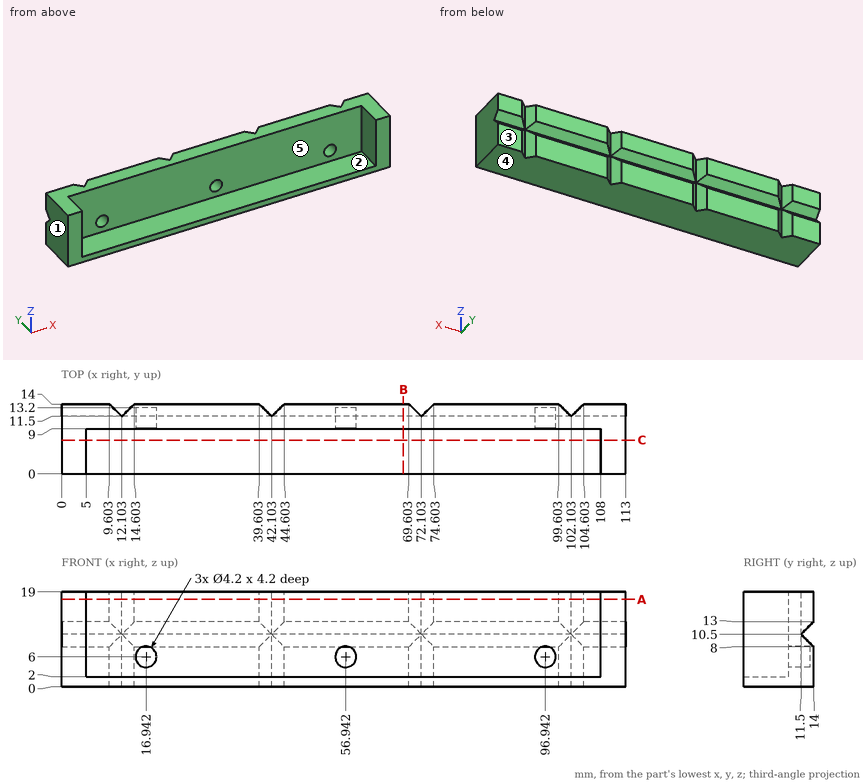
Print and shaded views of the part. All mm, measured from the part's lowest x, y and z. A direction names the side the tool comes from. Give positions to 0.01 mm unless a question says otherwise; leave off trailing zeros. Order: outer loops, then holes, each group sorted by start corner. A loop starts at its lowest first (then second) coordinate and runs counter-clockwise, first axis right, second up. Notation, with made-up numbers: (3.25, 79.5) - (8.25, 79.5) arc R8 cw to (8.25, 89.5) - close; hole circle Ø10 at (-9.5, 18.25). An arc over 180 degrees is marked (long way). One line per item, written item: value.
Item 1: Slice it at A-A (z = 17.5). List the corners of the cut face in (x, y), then the cut area to 3 significant figures.
Response values:
outline: (0, 0) - (5, 0) - (5, 9) - (108, 9) - (108, 0) - (113, 0) - (113, 14) - (104.6, 14) - (102.1, 11.5) - (99.6, 14) - (74.6, 14) - (72.1, 11.5) - (69.6, 14) - (44.6, 14) - (42.1, 11.5) - (39.6, 14) - (14.6, 14) - (12.1, 11.5) - (9.6, 14) - (0, 14) - close
area: 630 mm2
Item 2: Two-plate mould, pull along X, no slides. Class the marked faces 1, 2 and 3: released by +X, released by -X, zero draft, split by the parting line, or undercut.
Response values:
face 1: released by -X
face 2: undercut
face 3: zero draft
Item 3: Wall check: line 1 (X direction, y = 8.75, z = 16.5); line 2 (Z direction, x = 10, y = 2.75); line 3 (Y direction, x = 53.5, z = 5). Give the ranges that are in metal, low to high.
Response values:
line 1: 0 to 5, 108 to 113
line 2: 0 to 2
line 3: 9 to 14
Item 4: Tool access for the marked faces 4 and 5: list every direction of +Z, -Z, +X, -X, +Y, -Y with a clear straight run to the whole face (end or side of a thin tool).
Response values:
face 4: -Z, +X, -X, +Y, -Y
face 5: +Z, -Y
Item 5: Pin check, flat tips, straight feed: pin 1 Ø1.3 at (x, z) = (17.5, 6) entering from -Y; pin 2 Ø8.5 at (x, z) = (63.5, 13.5) entering from -Y. Stop position of each tip, or through.
Response values:
pin 1: y = 13.2
pin 2: y = 9
Item 6: Slice it at C-C (y = 6.75). List the corners of the cut face in (x, z).
Response values:
outline: (0, 0) - (113, 0) - (113, 19) - (108, 19) - (108, 2) - (5, 2) - (5, 19) - (0, 19) - close
Item 7: Slice it at B-B (x = 68.5). List the corners of the cut face in (y, z).
Response values:
outline: (0, 0) - (14, 0) - (14, 8) - (11.5, 10.5) - (14, 13) - (14, 19) - (9, 19) - (9, 2) - (0, 2) - close
